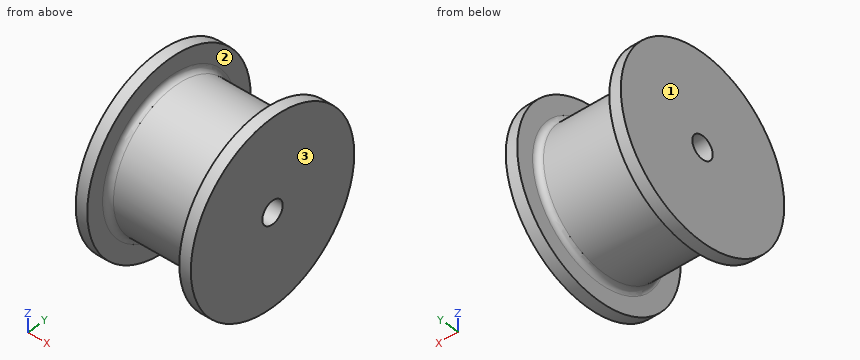
from build123d import *

# Parameters (mm, degrees)
F0_R          = 50.8
F1_DEPTH      = 31.75
F4_R          = 6.35
F5_DEPTH      = 31.751
F5_DEPTH_BACK = 31.751


with BuildPart() as f1:
    # F0 (on Right) → F1 (new body, symmetric)
    with BuildSketch(Plane.YZ):
        Circle(F0_R)
    extrude(amount=F1_DEPTH, both=True)

    # F2 (on Front) → F3 (revolve, cut)
    with BuildSketch(Plane.XZ):
        with BuildLine():
            ThreePointArc((25.4, 74.3732936617), (24.4700640303, 76.618357692), (22.225, 77.5482936617))
            Line((22.225, 77.5482936617), (-22.225, 77.5482936617))
            ThreePointArc((-22.225, 77.5482936617), (-24.4700640303, 76.618357692), (-25.4, 74.3732936617))
            Line((-25.4, 74.3732936617), (-25.4, 41.275))
            ThreePointArc((-25.4, 41.275), (-24.4700640303, 39.0299359697), (-22.225, 38.1))
            Line((-22.225, 38.1), (22.225, 38.1))
            ThreePointArc((22.225, 38.1), (24.4700640303, 39.0299359697), (25.4, 41.275))
            Line((25.4, 41.275), (25.4, 74.3732936617))
        make_face()
    revolve(axis=Axis((0, 0, 0), (1, 0, 0)), mode=Mode.SUBTRACT)

    # F4 (on Right) → F5 (cut, two sides)
    with BuildSketch(Plane.YZ) as f5_sk:
        Circle(F4_R)
    extrude(amount=-F5_DEPTH, mode=Mode.SUBTRACT)
    extrude(f5_sk.sketch, amount=F5_DEPTH_BACK, mode=Mode.SUBTRACT)


solid = f1.part
Could you check a few things on this model? Use its own coordinates, in mm. Face numbers are marked on the shaded views. Coordinates: 2 decimals unless noted, no trailing zeros. Order: outer loops, then holes, each group sorted by start corner. A loop starts at its lowest first (then second) coordinate and runs counter-clockwise, first axis right, second up. Notation, with made-up numbers: (48, 82) - (89, 82) arc R30 cw to (89, 119) - close; hole circle Ø2 at (65, -29.75). An arc over 180 degrees is marked (long way). Answer in a Markdown table with one row per item. Add a question column.
(1) If we mould it in two halves opening along X, with no side actions, what happens to the marked faces 1, 2 and 3? For each: released by +X, released by -X, zero draft, split by the parting line, or undercut.
(2) If we section it at C-C, the plane x = 19.5: Please give me the cut outline in (y, z), then the cut area to 3 significant figures.
(3) Will these pins go through, and if not, where does the flat tip stop? pin 1 (1 mm diameter, centred on x = -18.5, z = -29, fed in from -Y); pin 2 (5 mm diameter, centred on x = 17, z = -7.5, fed in from -Y); pin 3 (5 mm diameter, centred on x = -2.5, y = 5, fed in from +Z); pin 4 (16.5 mm diameter, centred on y = 0, z = 0, fed in from +X).
(4) If we section it at A-A, the plane z = 0: Please give me the cut outline in (x, y) (3 decimals), then the cut area to 3 significant figures.
(5) I need wall thicknesses on L1, parallel to Y at x = -18, z = 0; L2, parallel to X at y = 21, z = -44. Which ranges of each line are inside material? Lowest first, please.
Results are:
| question | item | result |
|---|---|---|
| 1 | face 1 | released by -X |
| 1 | face 2 | undercut |
| 1 | face 3 | released by +X |
| 2 | outline | circle Ø76.2 at (0, 0); hole circle Ø12.7 at (0, 0) |
| 2 | area | 4,430 mm2 |
| 3 | pin 1 | stops at y = -25.29 |
| 3 | pin 2 | stops at y = -37.77 |
| 3 | pin 3 | stops at z = 38.02 |
| 3 | pin 4 | stops at x = 31.75 |
| 4 | outline | (-31.75, -50.8) - (-25.4, -50.8) - (-25.4, -41.275) arc R3.175 cw to (-22.225, -38.1) - (22.225, -38.1) arc R3.175 cw to (25.4, -41.275) - (25.4, -50.8) - (31.75, -50.8) - (31.75, -6.35) - (-31.75, -6.35) - close; (-31.75, 6.35) - (31.75, 6.35) - (31.75, 50.8) - (25.4, 50.8) - (25.4, 41.275) arc R3.175 cw to (22.225, 38.1) - (-22.225, 38.1) arc R3.175 cw to (-25.4, 41.275) - (-25.4, 50.8) - (-31.75, 50.8) - close |
| 4 | area | 4,360 mm2 |
| 5 | L1 | y = -38.1 to -6.35, 6.35 to 38.1 |
| 5 | L2 | x = -31.75 to -25.4, 25.4 to 31.75 |
